Can you work these out from the model? Positions are in its coordinate system, mm. Face numbers are marked on the shaded views. Give positions to 0.01 mm unless a question says otherwise; leave off trailing zeros. Loops run counter-clockwise (first coordinate to the right, second up) from the corner with the lowest first, then second, coordinate; pieces in that order, holes last. Notation, with made-up numbers: (-23, 30) - (-14, 30) arc R13 cw to (-14, 35) - close; hole circle Ø3 at (23, 29). An arc over 180 degrees is marked (long way). Answer as a JSON object with one key per item and string values.
```python
from build123d import *

# Parameters (mm, degrees)
SKETCH2_W               = 630
SKETCH2_H               = 570
BOSS_EXTRUDE1_DEPTH     = 660
CUT_EXTRUDE1_DEPTH      = 928.213567632
CUT_EXTRUDE1_DEPTH_BACK = 928.213567632
SKETCH4_W               = 580
SKETCH4_H               = 610
CUT_EXTRUDE2_DEPTH      = 956.889637981
CUT_EXTRUDE2_DEPTH_BACK = 956.889637981
SKETCH5_W               = 520
SKETCH5_H               = 610


with BuildPart() as part:
    # Sketch2 → Boss-Extrude1 (new body)
    with BuildSketch(Plane(origin=(0, 0, 0), x_dir=(1, 0, 0), z_dir=(0, 1, 0))):
        Rectangle(SKETCH2_W, SKETCH2_H)
    extrude(amount=BOSS_EXTRUDE1_DEPTH)

    # Sketch4 → Cut-Extrude1 (cut, two sides: drawn at the far end of the back side and taken through both)
    with BuildSketch(Plane.XY.offset(285).offset(-CUT_EXTRUDE1_DEPTH_BACK)):
        with Locations((0, 330)):
            Rectangle(SKETCH4_W, SKETCH4_H)
    extrude(amount=CUT_EXTRUDE1_DEPTH + CUT_EXTRUDE1_DEPTH_BACK, mode=Mode.SUBTRACT)

    # Sketch5 → Cut-Extrude2 (cut, two sides: drawn at the far end of the back side and taken through both)
    with BuildSketch(Plane.ZY.offset(315).offset(-CUT_EXTRUDE2_DEPTH_BACK)):
        with Locations((0, 330)):
            Rectangle(SKETCH5_W, SKETCH5_H)
    extrude(amount=CUT_EXTRUDE2_DEPTH + CUT_EXTRUDE2_DEPTH_BACK, mode=Mode.SUBTRACT)


solid = part.part
```
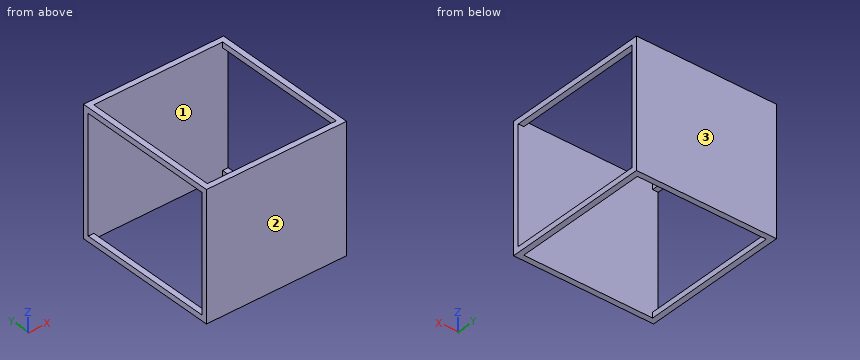
1) Imagine slicing it at B-B on y = 415. Write out the boundary of the cut face in (x, z).
Check sheet entries:
{"outline": "(-315, -285) - (-290, -285) - (-290, -260) - (-315, -260) - close; (-315, 260) - (-290, 260) - (-290, 285) - (-315, 285) - close; (290, -285) - (315, -285) - (315, -260) - (290, -260) - close; (290, 260) - (315, 260) - (315, 285) - (290, 285) - close"}
2) I need wall thicknesses on L1, parallel to Y at x = -164, z = 87.5. Which ranges of the line are inside material? Lowest first, please.
Check sheet entries:
{"L1": "0 to 25, 635 to 660"}
3) Imagine slicing it at A-A on x = 253. Write out the boundary of the cut face in (y, z), and give its area (3 significant figures).
Check sheet entries:
{"outline": "(0, -285) - (25, -285) - (25, 285) - (0, 285) - close; (635, -285) - (660, -285) - (660, 285) - (635, 285) - close", "area": "28,500 mm2"}
4) If we mould it in two halves opening along Y, with no side actions, what happens to the marked faces 1, 2 and 3? For each: released by +Y, released by -Y, zero draft, split by the parting line, or undercut.
Check sheet entries:
{"face 1": "undercut", "face 2": "released by -Y", "face 3": "released by +Y"}
5) Imagine slicing it at C-C on z = -249. Write out the boundary of the cut face in (x, y), and give its area (3 significant figures).
Check sheet entries:
{"outline": "(-315, 0) - (315, 0) - (315, 25) - (-315, 25) - close; (-315, 635) - (315, 635) - (315, 660) - (-315, 660) - close", "area": "31,500 mm2"}
